```python
from build123d import *

# Parameters (mm, degrees)
SKETCH_1_W          = 140
SKETCH_1_H          = 100
EXTRUDE_1_DEPTH     = 2
SKETCH_3_R          = 2.1
CUT_EXTRUDE_2_DEPTH = 10
CUT_EXTRUDE_3_DEPTH = 10
FILLET_1_R          = 5
FILLET_2_R          = 10


with BuildPart() as part:
    # 草图1 → 凸台-拉伸1 (new body)
    with BuildSketch(Plane.XY):
        Rectangle(SKETCH_1_W, SKETCH_1_H)
    extrude(amount=EXTRUDE_1_DEPTH)

    # 草图3 → 切除-拉伸2 (cut)
    with BuildSketch(Plane(origin=(0, 0, 0), x_dir=(-1, 0, 0), z_dir=(0, 0, -1))):
        with Locations((-15, -45)):
            Circle(SKETCH_3_R)
        with Locations((15, -45)):
            Circle(SKETCH_3_R)
        with Locations((15, 45)):
            Circle(SKETCH_3_R)
        with Locations((-15, 45)):
            Circle(SKETCH_3_R)
    extrude(amount=-CUT_EXTRUDE_2_DEPTH, mode=Mode.SUBTRACT)

    # 草图4 → 切除-拉伸3 (cut)
    with BuildSketch(Plane(origin=(0, 0, 0), x_dir=(-1, 0, 0), z_dir=(0, 0, -1))):
        Polygon((-17.5, 32.770587041), (-2.207059381, 0), (-17.5, -32.770587041), align=None)
        Polygon((-15.292940619, -37.5), (15.292940619, -37.5), (0, -4.729412959), align=None)
        Polygon((-15.292940619, 37.5), (15.292940619, 37.5), (0, 4.729412959), align=None)
        Polygon((17.5, -32.770587041), (17.5, 32.770587041), (2.207059381, 0), align=None)
        Polygon((-62.811364933, -45), (-45, -4.924428901), (-27.188635067, -45), align=None)
        Polygon((-65, -40.075571099), (-65, 40.075571099), (-47.188635067, 0), align=None)
        Polygon((-62.811364933, 45), (-27.188635067, 45), (-45, 4.924428901), align=None)
        Polygon((-25, -40.075571099), (-25, 40.075571099), (-42.811364933, 0), align=None)
        Polygon((42.811364933, 0), (25, 40.075571099), (25, -40.075571099), align=None)
        Polygon((45, -4.924428901), (27.188635067, -45), (62.811364933, -45), align=None)
        Polygon((45, 4.924428901), (27.188635067, 45), (62.811364933, 45), align=None)
        Polygon((65, -40.075571099), (47.188635067, 0), (65, 40.075571099), align=None)
    extrude(amount=-CUT_EXTRUDE_3_DEPTH, mode=Mode.SUBTRACT)

    # 圆角1
    fillet_1_edges = [part.edges().sort_by_distance(p)[0] for p in [
        (-62.811364933, 45, 1),
        (-45, 4.924428901, 1),
        (-27.188635067, 45, 1),
        (-65, 40.075571099, 1),
        (-65, -40.075571099, 1),
        (-47.188635067, 0, 1),
        (-45, -4.924428901, 1),
        (-62.811364933, -45, 1),
        (-27.188635067, -45, 1),
        (-2.207059381, 0, 1),
        (-17.5, 32.770587041, 1),
        (-17.5, -32.770587041, 1),
        (0, 4.729412959, 1),
        (15.292940619, 37.5, 1),
        (-15.292940619, 37.5, 1),
        (15.292940619, -37.5, 1),
        (0, -4.729412959, 1),
        (-15.292940619, -37.5, 1),
        (45, 4.924428901, 1),
        (62.811364933, 45, 1),
        (27.188635067, 45, 1),
        (65, 40.075571099, 1),
        (47.188635067, 0, 1),
        (65, -40.075571099, 1),
        (17.5, -32.770587041, 1),
        (17.5, 32.770587041, 1),
        (2.207059381, 0, 1),
        (-42.811364933, 0, 1),
        (-25, -40.075571099, 1),
        (-25, 40.075571099, 1),
        (27.188635067, -45, 1),
        (62.811364933, -45, 1),
        (45, -4.924428901, 1),
        (42.811364933, 0, 1),
        (25, 40.075571099, 1),
        (25, -40.075571099, 1),
    ]]
    fillet(fillet_1_edges, radius=FILLET_1_R)

    # 圆角2
    fillet_2_edges = [part.edges().sort_by_distance(p)[0] for p in [
        (-70, 50, 1),
        (70, 50, 1),
        (70, -50, 1),
        (-70, -50, 1),
    ]]
    fillet(fillet_2_edges, radius=FILLET_2_R)


solid = part.part
```
Source: CAD feature listing. Evaluate the final solid. Frame: model axes, mm. Round coordinates to 2 decimals unless told otherwise and drop trailing zeros. Loops run counter-clockwise (first coordinate to the right, second up) from the corner with the lowest first, then second, coordinate; pieces in that order, holes last.
1. Section query A-A on y = -24. Output: boundary loops of the cut face in (x, z), and give its area (3 significant figures).
2. Ray query, L1, parallel to Y at x = 42.5, z = 0.1; L2, parallel to Y at x = -45, z = 0.8; L3, parallel to Y at x = -11.5, z = 1.6. Return the intervals inside material, ascending.
3. Section query C-C on x = -15. Output: boundary loops of the cut face in (y, z).
4. Section query B-B on z = 1.7. Give the number of separate pieces and of enclosed holes in the cut face, and give its area (3 significant figures).
5. Mould query, pull axis X, two halves, no side actions, for faces 1 (the cylindrical face through (-67.15, 46.99, 1.01)), 2 (the cylindrical face through (30.652, -42.666, 1.014)). Classes: released by +X, released by -X, zero draft, split by the parting line, or undercut.
Answers below:
1. outline: (-70, 0) - (-53.48, 0) - (-53.48, 2) - (-70, 2) - close; (-36.52, 0) - (-8.99, 0) - (-8.99, 2) - (-36.52, 2) - close; (8.99, 0) - (36.52, 0) - (36.52, 2) - (8.99, 2) - close; (53.48, 0) - (70, 0) - (70, 2) - (53.48, 2) - close
1. area: 176 mm2
2. L1: y = -50 to -45, -12.91 to 12.91, 45 to 50
2. L2: y = -50 to -45, -12.24 to 12.24, 45 to 50
2. L3: y = -50 to -35.42, -29.37 to -15.13, 15.13 to 29.37, 35.42 to 50
3. outline: (-50, 0) - (-47.1, 0) - (-47.1, 2) - (-50, 2) - close; (-42.9, 0) - (-14.56, 0) - (-14.56, 2) - (-42.9, 2) - close; (14.56, 0) - (42.9, 0) - (42.9, 2) - (14.56, 2) - close; (47.1, 0) - (50, 0) - (50, 2) - (47.1, 2) - close
4. separate pieces: 1
4. enclosed holes: 16
4. area: 7,460 mm2
5. face 1: released by -X
5. face 2: undercut
